Geometry: see drawing. Coordinates: mm, zero at the bounding-box minimum. A direction names the side the tool comes from. Coordinates: 2 decimals unless noted, no trailing zeros. Loops run counter-clockwise (first coordinate to the right, second up) from the corner with the lowest first, then second, coordinate; pieces in that order, holes last. Notation, with made-up numbers: (73, -23.5) - (108, -23.5) arc R22 cw to (108, -2.5) - close; hole circle Ø8 at (-22, 22.5). An arc over 180 degrees is marked (long way). Write each question's results on one line, items separated by ' | '. Start each with the question number.
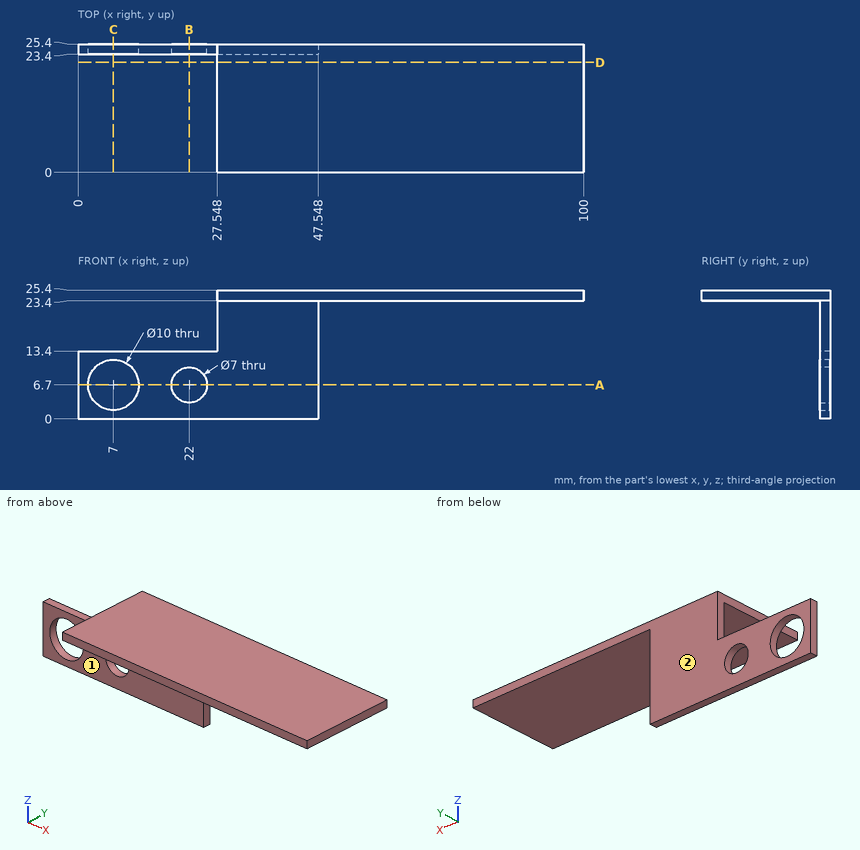
1) Section query B-B on x = 22. Output: boundary loops of the cut face in (y, z), and give its area (3 significant figures).
2) Section query D-D on y = 21.75. Output: boundary loops of the cut face in (x, z).
3) Access query for the marked faces 1 and 2. Directions: +Z, -Z, +X, -X, +Y, -Y. A direction counts if a zero-diameter tool reaches every point of the face in a straight line with its end or side. Return the directions, or none.
4) Pin query (flat end, axial travel): pin 1 Ø10 at (x, y) = (51.5, 18.5) entering from -Z; pin 2 Ø8 at (x, z) = (22, 6.7) entering from -Y; pin 3 Ø0.6 at (x, y) = (14, 24) entering from +Z; pin 4 Ø6 at (x, z) = (7, 6.7) entering from +Y. Return the tip coordinate at first contact, or that it passes through.
5) Section query A-A on z = 6.7. Output: boundary loops of the cut face in (x, y), and give its area (3 significant figures).
6) Section query C-C on x = 7. Output: boundary loops of the cut face in (y, z), and give its area (3 significant figures).
7) Material intervals for line 1 (X direction, y = 24.1, z = 6.7); line 2 (Z direction, x = 74.5, y = 13.5), sorted ascending. Write a range as [from, to].
Returned:
1) outline: (23.4, 0) - (25.4, 0) - (25.4, 3.2) - (23.4, 3.2) - close; (23.4, 10.2) - (25.4, 10.2) - (25.4, 13.4) - (23.4, 13.4) - close | area: 12.8 mm²
2) outline: (27.55, 23.4) - (100, 23.4) - (100, 25.4) - (27.55, 25.4) - close
3) face 1: -Z, +X, -X, -Y | face 2: +Z, -Z, +X, -X, +Y
4) pin 1: stops at z = 23.4 | pin 2: stops at y = 23.4 | pin 3: stops at z = 13.4 | pin 4: passes through
5) outline: (0, 23.4) - (2, 23.4) - (2, 25.4) - (0, 25.4) - close; (12, 23.4) - (18.5, 23.4) - (18.5, 25.4) - (12, 25.4) - close; (25.5, 23.4) - (47.55, 23.4) - (47.55, 25.4) - (25.5, 25.4) - close | area: 61.1 mm²
6) outline: (23.4, 0) - (25.4, 0) - (25.4, 1.7) - (23.4, 1.7) - close; (23.4, 11.7) - (25.4, 11.7) - (25.4, 13.4) - (23.4, 13.4) - close | area: 6.80 mm²
7) line 1: x = [0, 2], [12, 18.5], [25.5, 47.55] | line 2: z = [23.4, 25.4]
